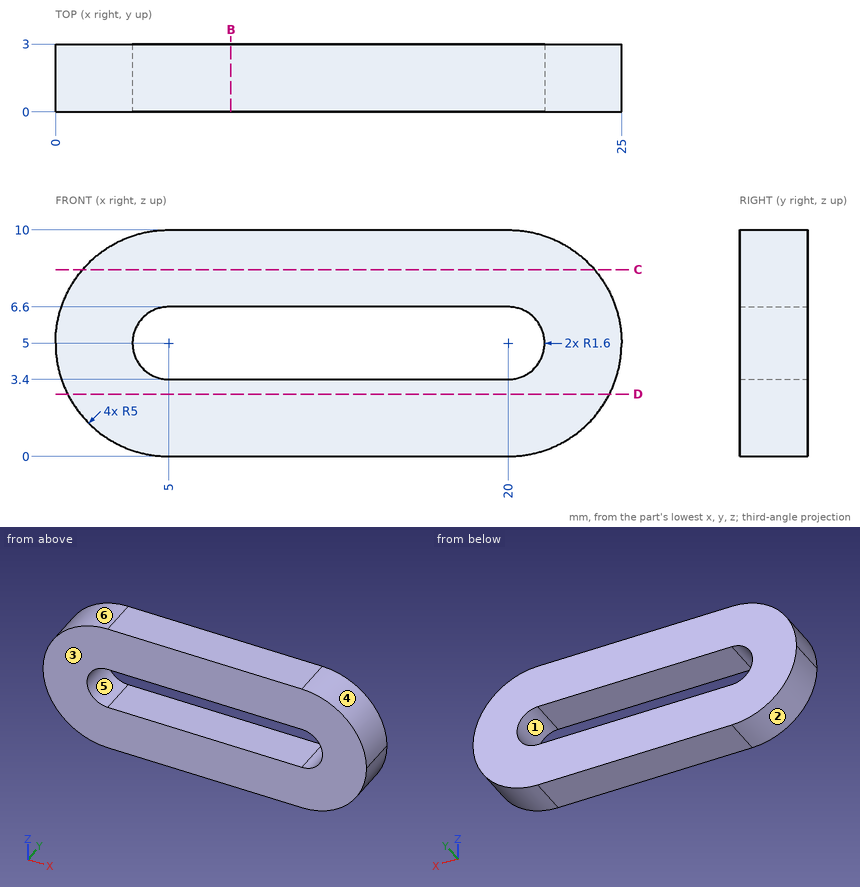
Answer from the drawing. Dimensions are ordinates in mm from the lowest x, y and z of the part. A direction names the side the tool comes from. Give positions to 0.01 mm unless a question says otherwise; leave off trailing zeros. Write each loop counter-clockwise with the first axis right and the second up, starting at its lowest first coordinate (ties: lowest second). Pieces come first, ordered by that corner, then holes. Notation, with made-up numbers: (85, -3.5) - (93, -3.5) arc R19 ccw to (93, 10.5) - close; hole circle Ø5 at (-38.75, -25). An arc over 180 degrees is marked (long way). Answer in a Markdown table with one row per item. Add a question column.
Item 1: Section C-C, the plane z = 8.25 is taken. Write down the section's boundary in (x, y).
Item 2: Section D-D, the plane z = 2.75 is taken. Write down the section's boundary in (x, y) (3 decimals), and give its area (3 significant figures).
Item 3: A flat-ended cylindrical pin translates along its axis: P1, Ø1.5, axis at y = 2, z = 6.5, coming from the -X side. Find the tip coordinate at first contact, or state that the pin passes through.
Item 4: Determine the mould class of the marked faces 3, 4, 5 and 6 for opening direction X: pulls with the +X half, pulls with the -X half, needs draft (parallel to the pull), parting line crosses it, or undercut.
Item 5: Section B-B, the plane x = 7.75 is taken. Write down the section's boundary in (y, z), and give its area (3 significant figures).
Item 6: Find the intervals of material crossed by L1, parallel to Z at x = 11.75, y = 1.3; L2, parallel to X at y = 0.4, z = 4; L3, parallel to X at y = 1.85, z = 1.25, in increasing order.
Item 7: A tool of negligible diameter and unlimited length cuts with its end or side. For the marked faces 1 and 2, from which of +Z, -Z, +X, -X, +Y, -Y can it reach the whole face along a straight path? Write none if from no direction.
Recorded:
| question | item | result |
|---|---|---|
| 1 | outline | (1.2, 0) - (23.8, 0) - (23.8, 3) - (1.2, 3) - close |
| 2 | outline | (0.535, 0) - (24.465, 0) - (24.465, 3) - (0.535, 3) - close |
| 2 | area | 71.8 mm2 |
| 3 | P1 | stops at x = 0.06 |
| 4 | face 3 | needs draft |
| 4 | face 4 | pulls with the +X half |
| 4 | face 5 | undercut |
| 4 | face 6 | pulls with the -X half |
| 5 | outline | (0, 0) - (3, 0) - (3, 3.4) - (0, 3.4) - close; (0, 6.6) - (3, 6.6) - (3, 10) - (0, 10) - close |
| 5 | area | 20.4 mm2 |
| 6 | L1 | z = 0 to 3.4, 6.6 to 10 |
| 6 | L2 | x = 0.1 to 3.75, 21.25 to 24.9 |
| 6 | L3 | x = 1.69 to 23.31 |
| 7 | face 1 | +Y, -Y |
| 7 | face 2 | -Z, -X, +Y, -Y |
